For this review, use the dimensioned drawing (mm, ordinates from the lowest corner) and the shaded views. Coordinates: 2 decimals unless noted, no trailing zeros. Order: outer loops, then holes, each group sorted by start corner. A loop starts at its lowest first (then second) coordinate and runs counter-clockwise, first axis right, second up. Notation, with made-up numbers: M 14.5,73 L 73.5,73 A22 ccw 73.5,110 Z; hole C 27,39 d10. An arc over 180 degrees is marked long. Answer as CSV lines item,"result". Start each with the question number.
Q1. Consider section D-D on z = 44. Write out the cut boundary in (x, y).
Q2. The part is to be moulded in two halves that separate along Y. For the marked faces 1, 2 and 3, say which applies: +Y half, -Y half, draft (parallel to the pull), parting line (faces both ways), or undercut.
Q3. For P1, Ø4, axis at x = 17, y = 19.5, coming from the +Z side, flat-tipped, find the tip position at first contact; note if it passes through.
Q4. Wall thickness on L1, parallel to Y at x = 20, z = 65; L2, parallel to Y at x = 20, z = 35; L3, parallel to X at y = 21, z = 42: over which ranges is each line inside the solid? List them lowest first. Write a range as [from, to].
Q5. Consider section B-B on x = 20. Write out the cut boundary in (y, z), and give its area (3 significant figures).
Q6. Consider section A-A on z = 69.5. Write out the cut boundary in (x, y).
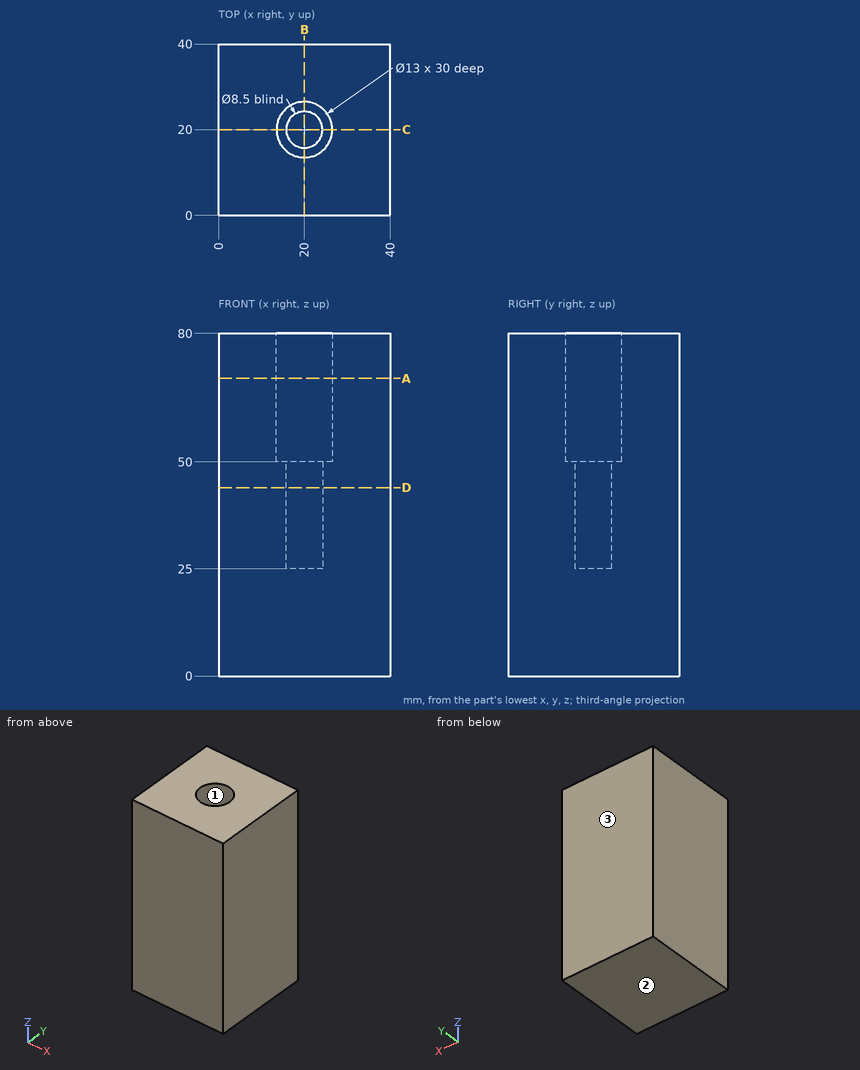
Evaluation:
1,outline,"M 0,0 L 40,0 L 40,40 L 0,40 Z; hole C 20,20 d8.5"
2,face 1,"undercut"
2,face 2,"draft"
2,face 3,"+Y half"
3,P1,"stops at z = 50"
4,L1,"y = [0, 13.5], [26.5, 40]"
4,L2,"y = [0, 15.75], [24.25, 40]"
4,L3,"x = [0, 15.87], [24.13, 40]"
5,outline,"M 0,0 L 40,0 L 40,80 L 26.5,80 L 26.5,50 L 24.25,50 L 24.25,25 L 15.75,25 L 15.75,50 L 13.5,50 L 13.5,80 L 0,80 Z"
5,area,"2,600 mm²"
6,outline,"M 0,0 L 40,0 L 40,40 L 0,40 Z; hole C 20,20 d13"
